The listing builds one solid part. Answer for the finished solid, in the listing's coordinates (mm). Face numbers are marked on the shaded views. A direction names the side the tool comes from. Coordinates: 2 decimals unless noted, no trailing zeros. Order: outer loops, then holes, each group sorted by start corner. A loop starts at its lowest first (then second) coordinate and runs counter-clockwise, first axis right, second up. Notation, with made-up numbers: (10.5, 69) -> (65.5, 69) arc R10 ccw to (65.5, 85) -> close; hole circle Ø11 at (8.25, 29). An arc over 180 degrees is marked (long way). Write each question's results on one line, items separated by ' | '. Start each with the question number.
(1) Straight lines are drawn through the part: L1, parallel to Y at x = -3, z = 229.5; L2, parallel to Z at x = -2.75, y = 2.5; L3, parallel to Y at x = -3, z = 220. For each, find the intervals that lie inside material, in ascending order.
(2) Given pin 1 (2 mm diameter, centred on x = -1, y = -8.5, fed in from +Z); pin 2 (4 mm diameter, centred on x = -3, z = 231.5, fed in from -Y); pin 3 (2.5 mm diameter, centred on x = -5, z = 216.5, fed in from -Y), each flat-ended and moving along its own axis, determine where each tip first touches the part or whether it passes through.
(3) The part is cut by section D-D, the plane z = 219.5. Give the vertices of the cut face in (x, y).
(4) Determine the mould class of the marked faces 1, 2 and 3 for opening direction Y: +Y half, -Y half, draft (parallel to the pull), parting line (faces both ways), or undercut.
(5) The part is cut by section A-A, the plane z = 229. Give the vertices of the cut face in (x, y), then the cut area to 3 significant figures.
(6) A tool of negligible diameter and unlimited length cuts with its end or side. For the marked faces 4, 5, 6, 7 and 8, from which of +Z, -Z, +X, -X, +Y, -Y can it reach the whole face along a straight path? Write none if from no direction.
(7) The part is cut by section C-C, the plane y = -21.5. Give the vertices of the cut face in (x, z), then the cut area to 3 significant figures.
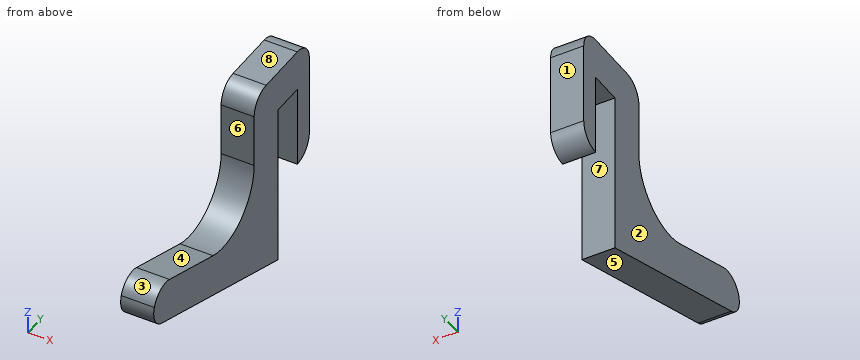
```python
from build123d import *

# Parameters (mm, degrees)
F1_DEPTH = 8
F2_R     = 4.99999
F3_R     = 13
F4_R     = 4.99999


# Not quite as in the source:
# - a fillet or chamfer is up to 0.001 mm smaller than in the source, because OpenCascade refuses the exact size


with BuildPart() as f1:
    # F0 (on Right) → F1 (new body)
    with BuildSketch(Plane.YZ):
        Polygon((11.3393977799, 240.6016960415), (-11.6606022201, 240.6016960415), (-11.6606022201, 204.5172253872), (-51.7021150763, 217.9898196767), (-54.8910993051, 208.5119306929), (-1.6606022201, 190.6016960415), (-1.6606022201, 230.6016960415), (6.3393977799, 230.6016960415), (6.3393977799, 210.6016960415), (11.3393977799, 210.6016960415), align=None)
    extrude(amount=-F1_DEPTH)

    # F2 (radius 5 in the source; OpenCascade refuses exactly that, so slightly less here)
    f2_edges = [f1.edges().sort_by_distance(p)[0] for p in [
        (-4, -51.702115, 217.98982),
        (-4, -54.891099, 208.511931),
    ]]
    fillet(f2_edges, radius=F2_R)

    # F3
    f3_edges = [f1.edges().sort_by_distance(p)[0] for p in [
        (-4, -11.660602, 204.517225),
    ]]
    fillet(f3_edges, radius=F3_R)

    # F4 (radius 5 in the source; OpenCascade refuses exactly that, so slightly less here)
    f4_edges = [f1.edges().sort_by_distance(p)[0] for p in [
        (-4, -11.660602, 240.601696),
        (-4, 11.339398, 240.601696),
        (-4, 11.339398, 210.601696),
    ]]
    fillet(f4_edges, radius=F4_R)


solid = f1.part
```
Established:
1) L1: y = -11.66 to -1.66, 6.34 to 11.34 | L2: z = 230.6 to 240.6 | L3: y = -11.92 to -1.66, 6.34 to 11.34
2) pin 1: stops at z = 240.53 | pin 2: stops at y = -11.66 | pin 3: stops at y = -52.03
3) outline: (-8, -12.04) -> (0, -12.04) -> (0, -1.66) -> (-8, -1.66) -> close; (-8, 6.34) -> (0, 6.34) -> (0, 11.34) -> (-8, 11.34) -> close
4) face 1: +Y half | face 2: draft | face 3: undercut
5) outline: (-8, -11.66) -> (0, -11.66) -> (0, -1.66) -> (-8, -1.66) -> close; (-8, 6.34) -> (0, 6.34) -> (0, 11.34) -> (-8, 11.34) -> close | area: 120 mm^2
6) face 4: +Z, +X, -X | face 5: -Z, +X, -X, -Y | face 6: +Z, +X, -X, -Y | face 7: -Z, +X, -X | face 8: +Z, +X, -X, +Y, -Y
7) outline: (-8, 197.28) -> (0, 197.28) -> (0, 210) -> (-8, 210) -> close | area: 102 mm^2
